Build history of the part. All positions in model axes, mm. A direction names the side the tool comes from. Give positions to 0.01 mm unless a question says otherwise; leave off trailing zeros. Loops run counter-clockwise (first coordinate to the right, second up) from the corner with the lowest first, then second, coordinate; pieces in that order, holes last. Notation, with made-up numbers: (-7.75, -17.5) - (42.25, -17.5) arc R20 cw to (42.25, 7.5) - close; hole circle Ø1 at (11.25, 15.5). An arc over 180 degrees is marked (long way). Return JSON: item names as keys, results as strings. Group by question number.
1) Slice it at C-C (x = -18). List the corners of the cut face in (y, z), and give its area (3 significant figures).
2) Slice it at A-A (y = -2). List the corners of the cut face in (x, z), and give its area (3 significant figures).
3) Drop flat-ended pins along their axis: pin 1 (3 mm diameter, centred on x = -27, z = 15, fed in from -Y); pin 2 (7.5 mm diameter, centred on x = 37, z = 17, fed in from +Y); pin 3 (13 mm diameter, centred on y = 7.5, z = 43, fed in from +X); pin 4 (21.5 mm diameter, centred on y = -4, z = 27, fed in from -X). Give the stop position or say it passes through.
4) Mould opens along X. For faces 4 (the face through (6, 22.96, 38)), 5 (the face through (30, -27, 82.55)), 6 (the face through (41.33, -3, 13)), 7 (the face through (-29.723, -3, 13)) say: released by +X, released by -X, zero draft, split by the parting line, or undercut.
5) 3-axis set-ups, long thin cutter, end or side, ignore diameter. For faces 1 (the face through (5, -3, 76.2)), 2 (the face through (-18, -27, 82.55)), 3 (the face through (5, -3, 0)): which of +Z, -Z, +X, -X, +Y, -Y reach the whole face in a straight line?
6) Slice it at D-D (z = 33.5). List the corners of the cut face in (x, y), and give its area (3 significant figures).
7) Slice it at B-B (z = 12.5). List the corners of the cut face in (x, y).
8) Drill centre lines: probe 1 along Z at (x, y) = (30.5, -0.5); probe 2 along Y at (x, z) = (-15, 9); probe 3 along Z at (x, y) = (34, 3). Where is each one in solid material? Low to high. Write a range as from..to.
```python
from build123d import *

# Parameters (mm, degrees)
F1_DEPTH = 82.55
F2_DEPTH = 76.2
F0_W     = 9.525
F0_H     = 19.05
F3_DEPTH = 25.4


# Not quite as in the source:
# - a feature of the source that left no trace in its solid (it failed there, or was rolled back) is left out
# - a pattern or mirror of a feature is missing from the dataset's text; its kind, count and spacing are read off the source's solid


with BuildPart() as f1:
    # F0 (on Top) → F1 (new body)
    with BuildSketch(Plane.XY):
        with BuildLine():
            ThreePointArc((-20.197500676, 18.3455366127), (-16.7326156752, 17.6181000932), (-14.7552827986, 20.5548919915))
            ThreePointArc((-14.7552827986, 20.5548919915), (-15.044803813, 21.8783314962), (-15.8604748841, 22.9599946804))
            ThreePointArc((-15.8604748841, 22.9599946804), (-20.234431152, 22.7256124785), (-20.197500676, 18.3455366127))
        make_face()
    extrude(amount=F1_DEPTH)

    # F1_copies: F1 across plane


with BuildPart() as f1b:
    # F0 (on Top) → F1, piece 2 (new body)
    with BuildSketch(Plane.XY):
        with BuildLine():
            ThreePointArc((32.7525223778, 20.5548919915), (30.9204110591, 23.4204148874), (27.5505643884, 22.9599946804))
            ThreePointArc((27.5505643884, 22.9599946804), (27.2638489298, 18.4265931888), (31.8045291463, 18.2994790273))
            ThreePointArc((31.8045291463, 18.2994790273), (32.5058902534, 19.3316198625), (32.7525223778, 20.5548919915))
        make_face()
    extrude(amount=F1_DEPTH)

    # F1_2_copies: F1b across plane


with BuildPart() as f1c:
    # F0 (on Top) → F1, piece 3 (new body)
    with BuildSketch(Plane.XY):
        with BuildLine():
            ThreePointArc((32.7651335661, -26.9655103104), (32.5151222308, -25.7316713922), (31.8045291463, -24.6924786227))
            ThreePointArc((31.8045291463, -24.6924786227), (27.3600452383, -24.7185591863), (27.3112643614, -29.1628519118))
            ThreePointArc((27.3112643614, -29.1628519118), (30.7800389767, -29.9054507611), (32.7651335661, -26.9655103104))
        make_face()
    extrude(amount=F1_DEPTH)

    # F1_3_copies: F1c across plane


with BuildPart() as f1d:
    # F0 (on Top) → F1, piece 4 (new body)
    with BuildSketch(Plane.XY):
        with BuildLine():
            ThreePointArc((-14.7564191649, -26.9655103104), (-16.7335847801, -24.0295514846), (-20.197500676, -24.7577854871))
            ThreePointArc((-20.197500676, -24.7577854871), (-20.1273922452, -29.2431839447), (-15.6421652409, -29.1628519118))
            ThreePointArc((-15.6421652409, -29.1628519118), (-14.9861867967, -28.150083675), (-14.7564191649, -26.9655103104))
        make_face()
    extrude(amount=F1_DEPTH)

    # F1_4_copies: F1d across plane


with BuildPart() as f1_1:
    add(f1.part)
    add(f1.part.mirror(Plane(origin=(0, 0, 38.1), x_dir=(-1, 0, 0), z_dir=(0, 0, -1))))



with BuildPart() as f1b_1:
    add(f1b.part)
    add(f1b.part.mirror(Plane(origin=(0, 0, 38.1), x_dir=(-1, 0, 0), z_dir=(0, 0, -1))))


with BuildPart() as f1c_1:
    add(f1c.part)
    add(f1c.part.mirror(Plane(origin=(0, 0, 38.1), x_dir=(-1, 0, 0), z_dir=(0, 0, -1))))


with BuildPart() as f1d_1:
    add(f1d.part)
    add(f1d.part.mirror(Plane(origin=(0, 0, 38.1), x_dir=(-1, 0, 0), z_dir=(0, 0, -1))))


with BuildPart() as f1_2:
    add(f1_1.part)

    add(f1b_1.part)  # F2 merges F1b

    add(f1c_1.part)  # F2 merges F1c

    add(f1d_1.part)  # F2 merges F1d
    # F0 (on Top) → F2 (join)
    with BuildSketch(Plane.XY):
        with BuildLine():
            ThreePointArc((-15.8604748841, 22.9599946804), (-15.044803813, 21.8783314962), (-14.7552827986, 20.5548919915))
            ThreePointArc((-14.7552827986, 20.5548919915), (-16.7326156752, 17.6181000932), (-20.197500676, 18.3455366127))
            Line((-20.197500676, 18.3455366127), (-20.197500676, 6.3188755628))
            Line((-20.197500676, 6.3188755628), (-20.197500676, -12.7311244372))
            Line((-20.197500676, -12.7311244372), (-20.197500676, -24.7577854871))
            ThreePointArc((-20.197500676, -24.7577854871), (-16.7335847801, -24.0295514846), (-14.7564191649, -26.9655103104))
            ThreePointArc((-14.7564191649, -26.9655103104), (-14.9861867967, -28.150083675), (-15.6421652409, -29.1628519118))
            Line((-15.6421652409, -29.1628519118), (27.3112643614, -29.1628519118))
            ThreePointArc((27.3112643614, -29.1628519118), (27.3600452383, -24.7185591863), (31.8045291463, -24.6924786227))
            Line((31.8045291463, -24.6924786227), (31.8045291463, -12.7214997977))
            Line((31.8045291463, -12.7214997977), (31.8045291463, 6.3285002023))
            Line((31.8045291463, 6.3285002023), (31.8045291463, 18.2994790273))
            ThreePointArc((31.8045291463, 18.2994790273), (27.2638489298, 18.4265931888), (27.5505643884, 22.9599946804))
            Line((27.5505643884, 22.9599946804), (-15.8604748841, 22.9599946804))
        make_face()
    extrude(amount=F2_DEPTH)

    # F0 (on Top) → F3 (join)
    with BuildSketch(Plane.XY):
        with Locations((-24.960000676, -3.2061244372)):
            Rectangle(F0_W, F0_H)
        with Locations((36.5670291463, -3.1964997977)):
            Rectangle(F0_W, F0_H)
    extrude(amount=F3_DEPTH)


solid = f1_2.part
```
Results:
{
 "1": {"outline": "(-30.13, -6.35) - (-23.8, -6.35) - (-23.8, 0) - (17.39, 0) - (17.39, -6.35) - (23.72, -6.35) - (23.72, 82.55) - (17.39, 82.55) - (17.39, 76.2) - (-23.8, 76.2) - (-23.8, 82.55) - (-30.13, 82.55) - close", "area": "4,260 mm2"},
 "2": {"outline": "(-29.72, 0) - (41.33, 0) - (41.33, 25.4) - (31.8, 25.4) - (31.8, 76.2) - (-20.2, 76.2) - (-20.2, 25.4) - (-29.72, 25.4) - close", "area": "4,450 mm2"},
 "3": {"pin 1": "y = -12.73", "pin 2": "y = 6.33", "pin 3": "x = 31.8", "pin 4": "x = -29.72"},
 "4": {"face 4": "undercut", "face 5": "zero draft", "face 6": "released by +X", "face 7": "released by -X"},
 "5": {"face 1": "+Z", "face 2": "+Z, +X, -X, +Y, -Y", "face 3": "-Z"},
 "6": {"outline": "(-20.2, -24.76) arc R3.17 ccw to (-15.64, -29.16) - (27.31, -29.16) arc R3.17 ccw (long way) to (31.8, -24.69) - (31.8, 18.3) arc R3.16 ccw to (27.55, 22.96) - (-15.86, 22.96) arc R3.17 ccw to (-20.2, 18.35) - close", "area": "2,730 mm2"},
 "7": {"outline": "(-29.72, -12.73) - (-20.2, -12.73) - (-20.2, -24.76) arc R3.17 ccw to (-15.64, -29.16) - (27.31, -29.16) arc R3.17 ccw (long way) to (31.8, -24.69) - (31.8, -12.72) - (41.33, -12.72) - (41.33, 6.33) - (31.8, 6.33) - (31.8, 18.3) arc R3.16 ccw to (27.55, 22.96) - (-15.86, 22.96) arc R3.17 ccw to (-20.2, 18.35) - (-20.2, 6.32) - (-29.72, 6.32) - close"},
 "8": {"probe 1": "0..76.2", "probe 2": "-29.16..22.96", "probe 3": "0..25.4"}
}
